The listing builds one solid part. Answer for the finished solid, in the listing's coordinates (mm). A direction names the side the tool comes from. Coordinates: 2 decimals unless noted, no trailing zeros. Loops run counter-clockwise (first coordinate to the right, second up) from the corner with the lowest first, then second, coordinate; pieces in that order, holes last. Notation, with made-up numbers: (78, 17) - (119, 17) arc R13 ccw to (119, 29) - close; hole circle Ø3 at (48, -30). An arc over 180 degrees is marked (long way). One line per question, with ' | ' between items.
from build123d import *

# Parameters (mm, degrees)
F1_DEPTH = 21.59
F2_R     = 3.81
F3_DEPTH = 0.508


with BuildPart() as f1:
    # F0 (on Front) → F1 (new body)
    with BuildSketch(Plane.XZ):
        with BuildLine():
            Line((-16.559356, -0.230847), (-16.051356, -0.230847))
            Line((-16.051356, -0.230847), (-16.051356, 10.011762))
            ThreePointArc((-16.051356, 10.011762), (-15.367777, 11.138266), (-14.052914, 11.052085))
            Line((-14.052914, 11.052085), (1.563488, 0.117363))
            Line((1.563488, 0.117363), (8.204864, 0.025492))
            ThreePointArc((8.204864, 0.025492), (9.4621, 0.546256), (9.982864, 1.803492))
            Line((9.982864, 1.803492), (9.982864, 12.546651))
            Line((9.982864, 12.546651), (9.474864, 12.546651))
            Line((9.474864, 12.546651), (9.474864, 1.803492))
            ThreePointArc((9.474864, 1.803492), (9.10289, 0.905467), (8.204864, 0.533492))
            Line((8.204864, 0.533492), (1.854864, 0.533492))
            Line((1.854864, 0.533492), (-13.761537, 11.468214))
            ThreePointArc((-13.761537, 11.468214), (-15.602345, 11.588867), (-16.559356, 10.011762))
            Line((-16.559356, 10.011762), (-16.559356, -0.230847))
        make_face()
    extrude(amount=F1_DEPTH)

    # F2 (on face) → F3 (cut, through all)
    with BuildSketch(Plane.YZ.offset(9.982864)):
        with Locations((-10.795, 7.466651)):
            Circle(F2_R)
    extrude(amount=-F3_DEPTH, mode=Mode.SUBTRACT)


solid = f1.part
Item 1: Each of these flat-tipped pins is pushed along its axis until it touches: pin 1 Ø6 at (x, y) = (-1, -9.5) entering from +Z; pin 2 Ø1 at (x, y) = (-1, -8.5) entering from -Z; pin 3 Ø1.5 at (x, y) = (4.5, -13) entering from +Z. Where does it stop, or does it pass through?
Taken from the geometry:
pin 1: stops at z = 4.63 | pin 2: stops at z = 1.56 | pin 3: stops at z = 0.53
Item 2: The mould has two halves that part along X. Classify faces 6 (the face through (-8, -21.59, 7)), 7 (the face through (9.983, -10.6, 3.5)), 8 (the face through (-16.559, -11, 5)), 9 (the face through (-6.35, -10.64, 5.66)): pulls with the +X half, pulls with the -X half, needs draft (parallel to the pull), parting line crosses it, or undercut.
Taken from the geometry:
face 6: needs draft | face 7: pulls with the +X half | face 8: pulls with the -X half | face 9: undercut
Item 3: Find the intervals of material crossed by line 1 (X direction, y = -11.75, z = 1.5); line 2 (X direction, y = -16, z = 3.75); line 3 (X direction, y = -11.75, z = 7), in increasing order. Write a range as [from, to].
Taken from the geometry:
line 1: x = [-16.56, -16.05], [-0.41, 0.47], [9.44, 9.96] | line 2: x = [-16.56, -16.05], [-3.62, -2.74], [9.47, 9.98] | line 3: x = [-16.56, -16.05], [-8.27, -7.38]
Item 4: Find section C-C, the plane z = 2.75. Write down the section's boundary in (x, y).
Taken from the geometry:
outline: (-16.56, -21.59) - (-16.05, -21.59) - (-16.05, 0) - (-16.56, 0) - close; (-2.2, -21.59) - (-1.31, -21.59) - (-1.31, 0) - (-2.2, 0) - close; (9.47, -21.59) - (9.98, -21.59) - (9.98, 0) - (9.47, 0) - close
Item 5: Find section A-A, the plane z = 4.5. Write down the section's boundary in (x, y).
Taken from the geometry:
outline: (-16.56, -21.59) - (-16.05, -21.59) - (-16.05, 0) - (-16.56, 0) - close; (-4.7, -21.59) - (-3.81, -21.59) - (-3.81, 0) - (-4.7, 0) - close; (9.47, -21.59) - (9.98, -21.59) - (9.98, -13.19) - (9.47, -13.19) - close; (9.47, -8.4) - (9.98, -8.4) - (9.98, 0) - (9.47, 0) - close
Item 6: Find section B-B, the plane y = -15.5. Write down the section's boundary in (x, z).
Taken from the geometry:
outline: (-16.56, -0.23) - (-16.05, -0.23) - (-16.05, 10.01) arc R1.27 cw to (-14.05, 11.05) - (1.56, 0.12) - (8.2, 0.03) arc R1.78 ccw to (9.98, 1.8) - (9.98, 12.55) - (9.47, 12.55) - (9.47, 1.8) arc R1.27 cw to (8.2, 0.53) - (1.85, 0.53) - (-13.76, 11.47) arc R1.78 ccw to (-16.56, 10.01) - close
Item 7: Which of the six approach directions +Z, -Z, +X, -X, +Y, -Y give full straight-line access (tool end or side, diameter ignored) to faces 1 (the face through (9.448, -10.644, 0.533)), 2 (the face through (-16.051, -11, 5)), 3 (the face through (9.73, -13.82, 5.15)), 4 (the face through (9.475, -8, 4)), 5 (the face through (-8, 0, 7))?
Taken from the geometry:
face 1: -Z, +X, +Y, -Y | face 2: -Z, +Y, -Y | face 3: +X | face 4: +Z, +Y, -Y | face 5: +Z, -Z, +X, -X, +Y
Item 8: Find section D-D, the plane y = -13. Write down the section's boundary in (x, z).
Taken from the geometry:
outline: (-16.56, -0.23) - (-16.05, -0.23) - (-16.05, 10.01) arc R1.27 cw to (-14.05, 11.05) - (1.56, 0.12) - (8.2, 0.03) arc R1.78 ccw to (9.98, 1.8) - (9.98, 4.36) - (9.47, 4.36) - (9.47, 1.8) arc R1.27 cw to (8.2, 0.53) - (1.85, 0.53) - (-13.76, 11.47) arc R1.78 ccw to (-16.56, 10.01) - close; (9.47, 10.57) - (9.98, 10.57) - (9.98, 12.55) - (9.47, 12.55) - close
